```python
from build123d import *

# Parameters (mm, degrees)
F1_DEPTH = 50
F2_W     = 81.249358
F2_H     = 37.196705
F3_DEPTH = 30


with BuildPart() as f1:
    # F0 (on Top) → F1 (new body)
    with BuildSketch(Plane.XY):
        with BuildLine():
            ThreePointArc((67.5, 20.704213), (0, 25.704213), (-67.5, 20.704213))
            Line((-67.5, 20.704213), (-67.5, -21.772621))
            Line((-67.5, -21.772621), (-45.624679, -21.772621))
            Line((-45.624679, -21.772621), (-45.624679, 14.025466))
            Line((-45.624679, 14.025466), (0, 14.025466))
            Line((0, 14.025466), (45.624679, 14.025466))
            Line((45.624679, 14.025466), (45.624679, -21.772621))
            Line((45.624679, -21.772621), (67.5, -21.772621))
            Line((67.5, -21.772621), (67.5, 20.704213))
        make_face()
    extrude(amount=F1_DEPTH)

    # F2 (on Front) → F3 (cut)
    with BuildSketch(Plane.XZ):
        with Locations((0, 11.401647)):
            Rectangle(F2_W, F2_H)
    extrude(amount=-F3_DEPTH, mode=Mode.SUBTRACT)


solid = f1.part
```
The model under review builds one solid part; all positions refer to its coordinate system, in mm. A direction names the side the tool comes from. Round coordinates to 2 decimals unless told otherwise and drop trailing zeros. Order: outer loops, then holes, each group sorted by start corner. A loop starts at its lowest first (then second) coordinate and runs counter-clockwise, first axis right, second up.
Item 1: Draft analysis for pull direction X (two halves, no side actions). For faces 1 (the cylindrical face through (0.948, 25.703, 30.206)), 2 (the flat face through (67.5, -1, 25)), 3 (the flat face through (-40.625, 19, 15)), 4 (the flat face through (-57, -21.773, 25)), state which applies: released by +X, released by -X, zero draft, split by the parting line, or undercut.
Working result:
face 1: split by the parting line
face 2: released by +X
face 3: undercut
face 4: zero draft
Item 2: Add section D-D, the plane z = 32. State the section outline as (x, y) points (3 decimals).
Working result:
outline: (-67.5, -21.773) - (-45.625, -21.773) - (-45.625, 14.025) - (45.625, 14.025) - (45.625, -21.773) - (67.5, -21.773) - (67.5, 20.704) arc R458.125 ccw to (-67.5, 20.704) - close
Item 3: To check wall thickness, follow probe 1 along X at (y, z) = (7, 24); probe 2 along Y at (x, z) = (-3, 42.5); probe 3 along X at (y, z) = (15, 16). State the ranges of each line that lie inside material, in increasing order.
Working result:
probe 1: x = -67.5 to -45.62, 45.62 to 67.5
probe 2: y = 14.03 to 25.69
probe 3: x = -67.5 to -40.62, 40.62 to 67.5
Item 4: For pin 1 (10 mm diameter, centred on x = -43.5, z = 30.5, fed in from -Y); pin 2 (12 mm diameter, centred on x = 8, y = 3.5, fed in from -Z); pin 3 (15 mm diameter, centred on x = -22.5, z = 36, fed in from -Y); pin 4 (13 mm diameter, centred on x = 13, y = 22.5, fed in from -Z), all flat-tipped, find the tip position at first contact; note any pin that passes through.
Working result:
pin 1: stops at y = -21.77
pin 2: passes through
pin 3: stops at y = 14.03
pin 4: stops at z = 30
Item 5: Machinability: for faces 5 (the flat face through (-45.625, -4, 25)), 6 (the flat face through (-67.5, 0, 25)), 7 (the flat face through (40.625, 19, 15)), which of the approach directions +Z, -Z, +X, -X, +Y, -Y give a long, thin tool a straight path to every point of the face, cutting with its end or side? Answer none if there is none.
Working result:
face 5: +Z, -Z, -Y
face 6: +Z, -Z, -X, +Y, -Y
face 7: -Z, +Y, -Y
Item 6: Add section A-A, the plane z = 7.5. State the section outline as (x, y) points (3 decimals), and give its area (3 significant figures).
Working result:
outline: (-67.5, -21.773) - (-45.625, -21.773) - (-45.625, 14.025) - (-40.625, 14.025) - (-40.625, 23.899) arc R458.125 ccw to (-67.5, 20.704) - close; (40.625, 14.025) - (45.625, 14.025) - (45.625, -21.773) - (67.5, -21.773) - (67.5, 20.704) arc R458.125 ccw to (40.625, 23.899) - close
area: 2,020 mm2
Item 7: Add section C-C, the plane y = 16. State the section outline as (x, z) points.
Working result:
outline: (-67.5, 0) - (-40.62, 0) - (-40.62, 30) - (40.62, 30) - (40.62, 0) - (67.5, 0) - (67.5, 50) - (-67.5, 50) - close
Item 8: Add section B-B, the plane y = 4.5. State the section outline as (x, z) points.
Working result:
outline: (-67.5, 0) - (-45.62, 0) - (-45.62, 50) - (-67.5, 50) - close; (45.62, 0) - (67.5, 0) - (67.5, 50) - (45.62, 50) - close
